```python
from build123d import *

# Parameters (mm, degrees)
SKETCH1_W                = 2.54
SKETCH1_H                = 2.54
BOSS_EXTRUDE1_DEPTH      = 2.5
BOSS_EXTRUDE2_DEPTH      = 6
BOSS_EXTRUDE2_DEPTH_BACK = 5.5
SKETCH2_W                = 0.65
SKETCH2_H                = 0.65
CHAMFER1_SIZE            = 0.2
CHAMFER2_SIZE            = 0.2


with BuildPart() as part:
    # Sketch1 → Boss-Extrude1 (new body)
    with BuildSketch(Plane(origin=(0, 0, 0), x_dir=(1, 0, 0), z_dir=(0, 1, 0))):
        Rectangle(SKETCH1_W, SKETCH1_H)
    extrude(amount=BOSS_EXTRUDE1_DEPTH)

    # Sketch2 → Boss-Extrude2 (add, two sides: drawn at the far end of the back side and taken through both)
    with BuildSketch(Plane(origin=(0, 2.5, 0), x_dir=(1, 0, 0), z_dir=(0, 1, 0)).offset(-BOSS_EXTRUDE2_DEPTH_BACK)):
        Rectangle(SKETCH2_W, SKETCH2_H)
    extrude(amount=BOSS_EXTRUDE2_DEPTH + BOSS_EXTRUDE2_DEPTH_BACK)

    # Chamfer1
    chamfer1_edges = [part.edges().sort_by_distance(p)[0] for p in [
        (1.27, 1.25, 1.27),
        (-1.27, 1.25, 1.27),
        (-1.27, 1.25, -1.27),
        (1.27, 1.25, -1.27),
    ]]
    chamfer(chamfer1_edges, length=CHAMFER1_SIZE)

    # Chamfer2
    chamfer2_edges = [part.edges().sort_by_distance(p)[0] for p in [
        (0.325, -3, 0),
        (0, -3, 0.325),
        (-0.325, -3, 0),
        (0, -3, -0.325),
        (0.325, 8.5, 0),
        (0, 8.5, -0.325),
        (-0.325, 8.5, 0),
        (0, 8.5, 0.325),
    ]]
    chamfer(chamfer2_edges, length=CHAMFER2_SIZE)


solid = part.part
```
The listing builds one solid part. Answer for the finished solid, in the listing's coordinates (mm). A direction names the side the tool comes from. Give positions to 0.01 mm unless a question says otherwise; leave off trailing zeros. Order: outer loops, then holes, each group sorted by start corner. A loop starts at its lowest first (then second) coordinate and runs counter-clockwise, first axis right, second up. Notation, with made-up numbers: (1.25, 77) - (59.25, 77) arc R33 cw to (59.25, 110) - close; hole circle Ø1 at (33.5, 25). An arc over 180 degrees is marked (long way). Use one line per item in the form item = value. Start each with the question number.
(1) For faces 1 (the flat face through (1, 0, 0)), 2 (the flat face through (1, 2.5, 0)), 3 (the flat face through (-1.27, 1, 0)), determine the directions among +Z, -Z, +X, -X, +Y, -Y from which every point of the face is accessible in a straight line to the end or side of a thin tool.
(2) Flat-ended cylindrical pins translate along their axes: pin 1 Ø0.7 at (y, z) = (4, 0) entering from -X (3 decimals); pin 2 Ø0.7 at (x, y) = (0, 5) entering from -Z (3 decimals); pin 3 Ø1.5 at (x, y) = (-0.5, 6.5) entering from +Z (3 decimals). Find the tip coordinate at first contact, or state that the pin passes through.
(3) A cutting plane is placed at B-B, the plane y = 3.25. Write down the section's boundary in (x, z) (3 decimals).
(4) Consider line 1 (Y direction, x = -0.65, z = 0.8); line 2 (X direction, y = -2, z = 0) (3 decimals). Determine where each line is inside the solid, lowest interval first. Write a range as from..to.
(5) A cutting plane is placed at A-A, the plane x = 0. Write down the section's boundary in (y, z) (3 decimals).
(6) A cutting plane is placed at C-C, the plane z = 0.85. Write down the section's boundary in (x, y).
Ans:
q1.face_1 = -Y
q1.face_2 = +Y
q1.face_3 = +Z, -Z, -X, +Y, -Y
q2.pin_1 = -0.325
q2.pin_2 = -0.325
q2.pin_3 = 0.325
q3.outline = (-0.325, -0.325) - (0.325, -0.325) - (0.325, 0.325) - (-0.325, 0.325) - close
q4.line_1 = 0..2.5
q4.line_2 = -0.325..0.325
q5.outline = (-3, -0.125) - (-2.8, -0.325) - (0, -0.325) - (0, -1.27) - (2.5, -1.27) - (2.5, -0.325) - (8.3, -0.325) - (8.5, -0.125) - (8.5, 0.125) - (8.3, 0.325) - (2.5, 0.325) - (2.5, 1.27) - (0, 1.27) - (0, 0.325) - (-2.8, 0.325) - (-3, 0.125) - close
q6.outline = (-1.27, 0) - (1.27, 0) - (1.27, 2.5) - (-1.27, 2.5) - close
